from build123d import *

# Parameters (mm, degrees)
SKETCH1_R            = 15.875
BOSS_EXTRUDE1_DEPTH  = 3.175
SKETCH5_W            = 3.175
SKETCH5_H            = 14.2875
BOSS_EXTRUDE3_DEPTH  = 76.2
CUT_EXTRUDE1_DEPTH   = 80.770887743
CIRPATTERN2_COUNT    = 4
BOSS_EXTRUDE21_DEPTH = 1.6002
SKETCH18_W           = 3.175
SKETCH18_H           = 7.9375
CUT_EXTRUDE7_DEPTH   = 7.9375
SKETCH19_W           = 15.875
SKETCH19_H           = 3.175
BOSS_EXTRUDE22_DEPTH = 7.9375
SKETCH20_R           = 4.7625
CUT_EXTRUDE8_DEPTH   = 106.553828833


with BuildPart() as part:
    # Sketch1 → Boss-Extrude1 (new body)
    with BuildSketch(Plane(origin=(0, 0, 0), x_dir=(0, 0, -1), z_dir=(1, 0, 0))):
        Circle(SKETCH1_R)
    extrude(amount=BOSS_EXTRUDE1_DEPTH)

    # Sketch5 → Boss-Extrude3 (add)
    with BuildSketch(Plane.ZY):
        with Locations((0, 7.14375)):
            Rectangle(SKETCH5_W, SKETCH5_H)
    boss_extrude3 = extrude(amount=BOSS_EXTRUDE3_DEPTH)

    # Sketch6 → Cut-Extrude1 (cut, symmetric)
    with BuildSketch(Plane.XY.offset(1.5875)):
        with BuildLine():
            Line((0, 14.2875), (-10.577102448, 14.2875))
            ThreePointArc((-10.577102448, 14.2875), (-9.60508653, 14.094154013), (-8.781051224, 13.543551224))
            Line((-8.781051224, 13.543551224), (-1.886948776, 6.649448776))
            ThreePointArc((-1.886948776, 6.649448776), (-1.06291347, 6.098845987), (-0.090897552, 5.9055))
            Line((-0.090897552, 5.9055), (0, 5.9055))
            Line((0, 5.9055), (0, 14.2875))
        make_face()
        with BuildLine():
            ThreePointArc((-67.291948776, 13.543551224), (-66.46791347, 14.094154013), (-65.495897552, 14.2875))
            Line((-65.495897552, 14.2875), (-76.2, 14.2875))
            Line((-76.2, 14.2875), (-76.2, 4.6355))
            Line((-76.2, 4.6355), (-67.291948776, 13.543551224))
        make_face()
    cut_extrude1 = extrude(amount=CUT_EXTRUDE1_DEPTH, both=True, mode=Mode.SUBTRACT)

    # CirPattern2: Boss-Extrude3, Cut-Extrude1 ×4 about axis
    cirpattern2_axis = Axis((0, 0, 0), (1, 0, 0))
    add([boss_extrude3.rotate(cirpattern2_axis, i * 360 / CIRPATTERN2_COUNT) for i in range(1, CIRPATTERN2_COUNT)])
    add([cut_extrude1.rotate(cirpattern2_axis, i * 360 / CIRPATTERN2_COUNT) for i in range(1, CIRPATTERN2_COUNT)], mode=Mode.SUBTRACT)

    # Sketch8 → Revolve1 (revolve)
    with BuildSketch(Plane.XY):
        Polygon((-76.2, 0), (-84.1248, 0), (-84.1248, 7.9375), (-76.2, 5.715), align=None)
    revolve(axis=Axis((0, 0, 0), (-1, 0, 0)))

    # Sketch17 → Boss-Extrude21 (add)
    with BuildSketch(Plane.ZY.offset(84.1248)):
        with BuildLine():
            Line((-7.9375, 0), (7.9375, 0))
            ThreePointArc((7.9375, 0), (0, -7.9375), (-7.9375, 0))
        make_face()
    extrude(amount=BOSS_EXTRUDE21_DEPTH)

    # Sketch18 → Cut-Extrude7 (cut, symmetric)
    with BuildSketch(Plane.XY):
        with Locations((-84.1375, 3.96875)):
            Rectangle(SKETCH18_W, SKETCH18_H)
    extrude(amount=CUT_EXTRUDE7_DEPTH, both=True, mode=Mode.SUBTRACT)

    # Sketch19 → Boss-Extrude22 (add, symmetric)
    with BuildSketch(Plane.XY):
        with Locations((-93.6625, 6.35)):
            Rectangle(SKETCH19_W, SKETCH19_H)
        Polygon((-85.725, 7.9375), (-82.55, 7.9375), (-82.55, 0), (-85.725, 0), (-85.725, 4.7625), align=None)
    extrude(amount=BOSS_EXTRUDE22_DEPTH, both=True)

    # Sketch20 → Cut-Extrude8 (cut, through all)
    with BuildSketch(Plane(origin=(0, 7.9375, 0), x_dir=(-1, 0, 0), z_dir=(0, 1, 0))):
        with BuildLine():
            ThreePointArc((101.6, 0), (99.275160076, -5.612660076), (93.6625, -7.9375))
            Line((93.6625, -7.9375), (101.6, -7.9375))
            Line((101.6, -7.9375), (101.6, 0))
        make_face()
        with BuildLine():
            ThreePointArc((93.6625, 7.9375), (99.275160076, 5.612660076), (101.6, 0))
            Line((101.6, 0), (101.6, 7.9375))
            Line((101.6, 7.9375), (93.6625, 7.9375))
        make_face()
        with Locations(Location((93.6625, 0, 0), (0, 0, 90))):
            Circle(SKETCH20_R)
    extrude(amount=-CUT_EXTRUDE8_DEPTH, mode=Mode.SUBTRACT)


solid = part.part
The listing builds one solid part. Answer for the finished solid, in the listing's coordinates (mm). A direction names the side the tool comes from. Give positions to 0.01 mm unless a question says otherwise; leave off trailing zeros. Order: outer loops, then holes, each group sorted by start corner. A loop starts at its lowest first (then second) coordinate and runs counter-clockwise, first axis right, second up. Notation, with made-up numbers: (71.25, 7) -> (101.25, 7) arc R10 ccw to (101.25, 17) -> close; hole circle Ø1 at (36, 52.25). An arc over 180 degrees is marked (long way). Put each result on its own line as item: value.
Item 1: A cutting plane is placed at B-B on x = -40. Give the vertices of the cut face in (y, z), plus the area to 3 significant figures.
Established:
outline: (-14.29, -1.59) -> (-1.59, -1.59) -> (-1.59, -14.29) -> (1.59, -14.29) -> (1.59, -1.59) -> (14.29, -1.59) -> (14.29, 1.59) -> (1.59, 1.59) -> (1.59, 14.29) -> (-1.59, 14.29) -> (-1.59, 1.59) -> (-14.29, 1.59) -> close
area: 171 mm^2
Item 2: A cutting plane is placed at A-A on z = 11. Give the vertices of the cut face in (x, y) (1 decimal).
Established:
outline: (-69.8, -1.6) -> (-6.2, -1.6) -> (-6.2, 1.6) -> (-69.8, 1.6) -> close; (0, -11.4) -> (3.2, -11.4) -> (3.2, 11.4) -> (0, 11.4) -> close
Item 3: For faces 4 (the face through (-38, -8, -1.587)), 5 (the face through (-38, 8, -1.588)), 6 (the face through (-5.38, -10.14, 0.02)), 7 (the face through (-88, 4.762, 0)), determine the directions among +Z, -Z, +X, -X, +Y, -Y from which every point of the face is accessible in a straight line to the end or side of a thin tool.
Established:
face 4: -Z, -Y
face 5: -Z, +Y
face 6: +Z, -Z, -Y
face 7: +Z, -Z, -X, -Y
Item 4: Given P1, Ø17.5, axis at x = -93.5, z = -3.5, coming from the -Y side; P2, Ø14, axis at x = -42, y = 7.5, coming from the -Z side; P3, Ø1.5, axis at x = -54, z = 9, coming from the +Y side, each flat-ended and moving along its own axis, determine where each tip first touches the part or whether it passes through.
Established:
P1: stops at y = -7.94
P2: stops at z = -14.29
P3: stops at y = 1.59
Item 5: Straight lines are drawn through the part: line 1 (Z direction, x = -13, y = 4); line 2 (X direction, y = 4, z = -12.5) (3 decimals). For each, find the intervals that lie inside material, in ascending order.
Established:
line 1: z = -1.59 to 1.59
line 2: x = 0 to 3.175
Item 6: For a pull along X with two mould halves and no side action, classify faces 1 (the face through (-9.62, -0.02, -14.1)), 2 (the face through (1.565, -15.497, 3.441)), 3 (the face through (-66.48, 0.02, -14.09)) as released by +X, released by -X, zero draft, split by the parting line, or undercut.
Established:
face 1: undercut
face 2: zero draft
face 3: released by -X
